from build123d import *

# Parameters (mm, degrees)
SKETCH_W             = 90
SKETCH_H             = 35
PAD_DEPTH            = 15
SKETCH001_R          = 2
PAD001_DEPTH         = 10
FILLET_R             = 2
FILLET001_R          = 3
FILLET002_R          = 1
BODY_PLACEMENT_ANGLE = 90


with BuildPart() as part:
    # Sketch → Pad (new body, symmetric)
    with BuildSketch(Plane.XY):
        Rectangle(SKETCH_W, SKETCH_H)
    extrude(amount=PAD_DEPTH, both=True)

    # Sketch001 (on Face4 of Pad) → Pad001 (join)
    with BuildSketch(Plane(origin=(-45, 0, 0), x_dir=(0, -1, 0), z_dir=(-1, 0, 0))):
        with Locations((-8.41, 10.070301)):
            Circle(SKETCH001_R)
        with Locations((-8.41, -10.070301)):
            Circle(SKETCH001_R)
    extrude(amount=PAD001_DEPTH)

    # Fillet
    fillet_edges = [part.edges().sort_by_distance(p)[0] for p in [
        (-45, 17.5, 0),
        (45, 17.5, 0),
        (0, 17.5, -15),
        (0, 17.5, 15),
    ]]
    fillet(fillet_edges, radius=FILLET_R)

    # Fillet001
    fillet001_edges = [part.edges().sort_by_distance(p)[0] for p in [
        (45, -17.5, 0),
        (-45, -17.5, 0),
        (0, -17.5, -15),
        (0, -17.5, 15),
    ]]
    fillet(fillet001_edges, radius=FILLET001_R)

    # Fillet002
    fillet002_edges = [part.edges().sort_by_distance(p)[0] for p in [
        (-45, 0.5, -15),
        (-45, 0.5, 15),
        (45, 0.5, 15),
        (45, 0.5, -15),
    ]]
    fillet(fillet002_edges, radius=FILLET002_R)


with BuildPart() as part_1:
    # Body placement: moved
    add(part.part.moved(Location((0, 0, 23))).rotate(Axis((0, 0, 23), (1, 0, 0)), BODY_PLACEMENT_ANGLE))


solid = part_1.part
CAD build for the part. Positions are in the model's coordinates, mm. A direction names the side the tool comes from. Give positions to 0.01 mm unless a question says otherwise; leave off trailing zeros. Write each loop counter-clockwise with the first axis right and the second up, starting at its lowest first coordinate (ties: lowest second). Pieces come first, ordered by that corner, then holes. Notation, with made-up numbers: (-4.75, 56) - (52.25, 56) arc R22 cw to (52.25, 93) - close; hole circle Ø8 at (62, 82.5). An arc over 180 degrees is marked (long way). Answer as CSV lines item,"result".
Q1. Band-saw the part on D-D (y = -11). Give the cut face in (x, z).
Result set:
outline,"(-55, 29.64) - (-45, 29.64) - (-45, 8.5) arc R3 ccw to (-42, 5.5) - (42, 5.5) arc R3 ccw to (45, 8.5) - (45, 38.5) arc R2 ccw to (43, 40.5) - (-43, 40.5) arc R2 ccw to (-45, 38.5) - (-45, 33.18) - (-55, 33.18) - close"
Q2. Band-saw the part on B-B (y = -4). Give the cut face in (x, z).
Result set:
outline,"(-45, 8.5) arc R3 ccw to (-42, 5.5) - (42, 5.5) arc R3 ccw to (45, 8.5) - (45, 38.5) arc R2 ccw to (43, 40.5) - (-43, 40.5) arc R2 ccw to (-45, 38.5) - close"
Q3. Band-saw the part on A-A (z = 17). Give the cut face in (x, y), and give its area (3 significant figures).
Result set:
outline,"(-45, -14) arc R1 ccw to (-44, -15) - (44, -15) arc R1 ccw to (45, -14) - (45, 14) arc R1 ccw to (44, 15) - (-44, 15) arc R1 ccw to (-45, 14) - close"
area,"2,700 mm²"
Q4. 3-axis set-ups, long thin cutter, end or side, ignore diameter. For faces 1 (the face through (44.1, -0.2, 6.36)), 2 (the face through (-49.93, 8.087, 31.67)): which of +Z, -Z, +X, -X, +Y, -Y reach the whole face in a straight line?
Result set:
face 1,"-Z, +X, +Y, -Y"
face 2,"-X"
Q5. Drill centre lines: line 1 (X direction, y = -5.5, z = 32.5); line 2 (X direction, y = 13, z = 39). Where is each one in solid material? Low to high. Write a range as from..to.
Result set:
line 1,"-45..45"
line 2,"-44.94..44.94"
Q6. Pull direction Y, two halves, no side cores. Call faces 3 (the face through (0.62, -14.1, 6.36)), 4 (the face through (-49.93, -8.296, 30.487)), 5 (the face through (45, 0, 23)): released by +Y, released by -Y, zero draft, split by the parting line, or undercut.
Result set:
face 3,"released by -Y"
face 4,"undercut"
face 5,"zero draft"
Q7. Band-saw the part on C-C (z = 31.41). Give the cut face in (x, y).
Result set:
outline,"(-55, -12.07) - (-45, -12.07) - (-45, -14) arc R1 ccw to (-44, -15) - (44, -15) arc R1 ccw to (45, -14) - (45, 14) arc R1 ccw to (44, 15) - (-44, 15) arc R1 ccw to (-45, 14) - (-45, 12.07) - (-55, 12.07) - (-55, 8.07) - (-45, 8.07) - (-45, -8.07) - (-55, -8.07) - close"
